Work out the finished part from the listing and answer in its coordinate system (mm). A direction names the side the tool comes from. Round coordinates to 2 decimals unless told otherwise and drop trailing zeros. Loops run counter-clockwise (first coordinate to the right, second up) from the corner with the lowest first, then second, coordinate; pieces in that order, holes last. Notation, with made-up numbers: M 63,65.5 L 98,65.5 A7 cw 98,69.5 Z; hole C 3,-8 d8. An arc over 180 degrees is marked long. One line per item, written item: value.
```python
from build123d import *

# Parameters (mm, degrees)
PAD_DEPTH       = 3
SKETCH001_W     = 7
SKETCH001_H     = 2.5
PAD001_DEPTH    = 7
SKETCH002_R     = 2.125
POCKET_DEPTH    = 2.5
FILLET_R        = 3.49
FILLET001_R     = 3.5
FILLET002_R     = 1
SKETCH003_R     = 1.25
POCKET001_DEPTH = 25


with BuildPart() as part:
    # Sketch → Pad (new body)
    with BuildSketch(Plane.XZ):
        Polygon((0, 0), (0, 5), (15, 5), (15, 35), (80, 35), (80, 5), (150, 5), (150, 0), align=None)
    extrude(amount=PAD_DEPTH)

    # Sketch001 (on Face9 of Pad) → Pad001 (join)
    with BuildSketch(Plane(origin=(0, 0, 0), x_dir=(1, 0, 0), z_dir=(0, 1, 0))):
        with Locations((3.5, -3.75)):
            Rectangle(SKETCH001_W, SKETCH001_H)
    extrude(amount=PAD001_DEPTH)

    # Sketch002 (on Face9 of Pad001) → Pocket (cut)
    with BuildSketch(Plane(origin=(0, 0, 5), x_dir=(-1, 0, 0), z_dir=(0, 0, 1))):
        with Locations((-3.5, -3.5)):
            Circle(SKETCH002_R)
    extrude(amount=-POCKET_DEPTH, mode=Mode.SUBTRACT)

    # Fillet
    fillet_edges = [part.edges().sort_by_distance(p)[0] for p in [
        (0, 7, 3.75),
        (7, 7, 3.75),
    ]]
    fillet(fillet_edges, radius=FILLET_R)

    # Fillet001
    fillet001_edges = [part.edges().sort_by_distance(p)[0] for p in [
        (15, -1.5, 35),
        (15, -1.5, 5),
        (80, -1.5, 5),
        (80, -1.5, 35),
    ]]
    fillet(fillet001_edges, radius=FILLET001_R)

    # Fillet002
    fillet002_edges = [part.edges().sort_by_distance(p)[0] for p in [
        (150, -1.5, 5),
        (150, -1.5, 0),
    ]]
    fillet(fillet002_edges, radius=FILLET002_R)

    # Sketch003 (on Face13 of Fillet) → Pocket001 (cut)
    with BuildSketch(Plane.XZ.offset(3)):
        with Locations((18.5, 31.5)):
            Circle(SKETCH003_R)
        with Locations((18.5, 8.5)):
            Circle(SKETCH003_R)
        with Locations((76.5, 8.5)):
            Circle(SKETCH003_R)
        with Locations((76.5, 31.5)):
            Circle(SKETCH003_R)
    extrude(amount=-POCKET001_DEPTH, mode=Mode.SUBTRACT)


solid = part.part
```
1) For faces 5 (the face through (47, -1, 35)), 6 (the face through (3, 1, 2.5)), 7 (the face through (116, -1, 5)), determine the directions among +Z, -Z, +X, -X, +Y, -Y from which every point of the face is accessible in a straight line to the end or side of a thin tool.
Check values:
face 5: +Z, +X, -X, +Y, -Y
face 6: -Z, +X, -X, +Y
face 7: +Z, +X, +Y, -Y
2) Find section A-A (x = 135). Give the vertices of the cut face in (y, z).
Check values:
outline: M -3,0 L 0,0 L 0,5 L -3,5 Z
3) The mould has two halves that part along X. Classify faces 1 (the face through (77.69, -1.52, 31.88)), 2 (the face through (5.19, 4.79, 3.77)), 3 (the face through (15, -1, 20)), 4 (the face through (7, 2, 4)): +X half, -X half, draft (parallel to the pull), parting line (faces both ways), or undercut.
Check values:
face 1: undercut
face 2: undercut
face 3: -X half
face 4: +X half
4) Find the intervals of material crossed by probe 1 along Z at (x, y) = (76.5, -2.2); probe 2 along X at (y, z) = (3.5, 3.8) (3 decimals); probe 3 along Y at (x, z) = (3.5, 3.65) (3 decimals), in increasing order. Write a range as from..to.
Check values:
probe 1: 0..7.25, 9.75..30.25, 32.75..35
probe 2: 0..1.375, 5.625..7
probe 3: -3..1.375, 5.625..7
5) Each of these flat-tipped pins is pushed along its axis until it touches: pin 1 (1.5 mm diameter, centred on x = 104, y = -1.5, fed in from +Z); pin 2 (1.2 mm diameter, centred on y = 1.5, z = 4, fed in from +X); pin 3 (6 mm diameter, centred on y = -2, z = 30.5, fed in from +X). Where does it stop, or does it pass through?
Check values:
pin 1: z = 5
pin 2: x = 7
pin 3: x = 80
6) Find section B-B (z = 21). Give the vertices of the cut face in (x, y).
Check values:
outline: M 15,-3 L 80,-3 L 80,0 L 15,0 Z
